The drawing under review shows one solid part. Ordinate dimensions are in mm from its lowest x, y, z. A direction names the side the tool comes from. Coordinates: 2 decimals unless noted, no trailing zeros. Write each loop counter-clockwise with the first axis right and the second up, starting at its lowest first coordinate (ties: lowest second). Pieces come first, ordered by that corner, then holes. Notation, with made-up numbers: (64.25, 66.5) - (112.25, 66.5) arc R19 cw to (112.25, 77.5) - close; hole circle Ø9 at (-21, -39). An arc over 180 degrees is marked (long way). Use a Markdown table: item, result.
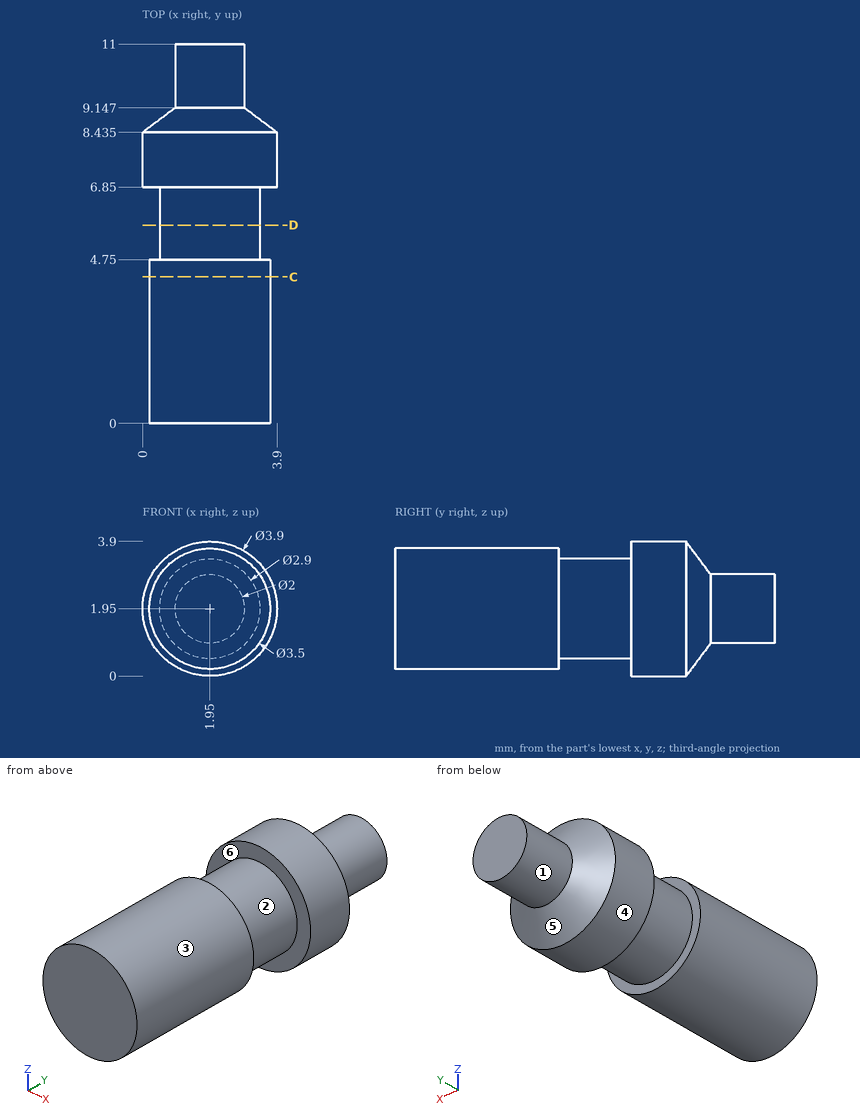
(1) Take a section at D-D on y = 5.75. Write out the cut boundary in (x, z).
Determined:
| item | result |
|---|---|
| outline | circle Ø2.9 at (1.95, 1.95) |
(2) Machinability: for the marked faces 1, 2 and 3, which of the approach directions +Z, -Z, +X, -X, +Y, -Y give a long, thin tool a straight path to every point of the face, cutting with its end or side? Answer none if there is none.
Determined:
| item | result |
|---|---|
| face 1 | +Y |
| face 2 | none |
| face 3 | -Y |
(3) Draft analysis for pull direction Y (two halves, no side actions). For the marked faces 4, 5 and 6, state which applies: +Y half, -Y half, draft (parallel to the pull), parting line (faces both ways), or undercut.
Determined:
| item | result |
|---|---|
| face 4 | draft |
| face 5 | +Y half |
| face 6 | undercut |
(4) For pin 1 (1.5 mm diameter, centred on x = 3, y = 8.5, fed in from -Z), flat-tipped, find the tip position at first contact; note if it passes through.
Determined:
| item | result |
|---|---|
| pin 1 | z = 0.02 |
(5) Take a section at C-C on y = 4.25. Write out the cut boundary in (x, z).
Determined:
| item | result |
|---|---|
| outline | circle Ø3.5 at (1.95, 1.95) |
(6) For L1, parallel to Y at x = 0.9, z = 0.7; L2, parallel to Y at x = 0.85, z = 3.5; L3, parallel to X at y = 3.5, z = 2.15, list the stretches that pass through material, from the lowest coordinate up. Write a range as from..to.
Determined:
| item | result |
|---|---|
| L1 | 0..4.75, 6.85..8.67 |
| L2 | 6.85..8.47 |
| L3 | 0.21..3.69 |
